The model under review builds one solid part; all positions refer to its coordinate system, in mm. A direction names the side the tool comes from. Give positions to 0.01 mm unless a question says otherwise; leave off trailing zeros. Loops run counter-clockwise (first coordinate to the right, second up) from the corner with the lowest first, then second, coordinate; pieces in that order, holes last. Notation, with made-up numbers: M -15.5,-24 L 13.5,-24 A18 cw 13.5,-17 Z; hole C -24,32.25 d7. An arc over 180 degrees is marked long. Return JSON: item names as keys, results as strings.
```python
from build123d import *

# Parameters (mm, degrees)
SKETCH1_W           = 320
SKETCH1_H           = 82.5
BOSS_EXTRUDE1_DEPTH = 43.48
SKETCH3_W           = 20
SKETCH3_H           = 20
CUT_EXTRUDE1_DEPTH  = 15
SKETCH5_W           = 320
SKETCH5_H           = 82.5
BOSS_EXTRUDE3_DEPTH = 5


with BuildPart() as part:
    # Sketch1 → Boss-Extrude1 (new body)
    with BuildSketch(Plane(origin=(0, 0, 0), x_dir=(1, 0, 0), z_dir=(0, 1, 0))):
        Rectangle(SKETCH1_W, SKETCH1_H)
        Polygon((-135, 30), (-115, 30), (-115, 7.5), (-10, 7.5), (-10, 30), (10, 30), (10, 7.5), (115, 7.5), (115, 30), (135, 30), (135, -30), (115, -30), (115, -7.5), (10, -7.5), (10, -30), (-10, -30), (-10, -7.5), (-115, -7.5), (-115, -30), (-135, -30), align=None, mode=Mode.SUBTRACT)
    extrude(amount=-BOSS_EXTRUDE1_DEPTH)

    # Sketch3 → Cut-Extrude1 (cut)
    with BuildSketch(Plane.XY.offset(41.25)):
        with Locations((0, -33.48)):
            Rectangle(SKETCH3_W, SKETCH3_H)
        with Locations((125, -33.48)):
            Rectangle(SKETCH3_W, SKETCH3_H)
        with Locations((-125, -33.48)):
            Rectangle(SKETCH3_W, SKETCH3_H)
    extrude(amount=-CUT_EXTRUDE1_DEPTH, mode=Mode.SUBTRACT)

    # Sketch5 → Boss-Extrude3 (add)
    with BuildSketch(Plane.XZ.offset(43.48)):
        Rectangle(SKETCH5_W, SKETCH5_H)
    extrude(amount=BOSS_EXTRUDE3_DEPTH)


solid = part.part
```
1) Consider section A-A on y = -38.5. Write out the cut boundary in (x, z).
From the geometry:
{"outline": "M -160,-41.25 L 160,-41.25 L 160,41.25 L 135,41.25 L 135,-30 L 115,-30 L 115,-7.5 L 10,-7.5 L 10,-30 L -10,-30 L -10,-7.5 L -115,-7.5 L -115,-30 L -135,-30 L -135,41.25 L -160,41.25 Z; M -115,7.5 L -10,7.5 L -10,41.25 L -115,41.25 Z; M 10,7.5 L 115,7.5 L 115,41.25 L 10,41.25 Z"}
2) Consider section C-C on x = 4.5. Write out the cut boundary in (y, z), then the cut area to 3 significant figures.
From the geometry:
{"outline": "M -48.48,-41.25 L 0,-41.25 L 0,-30 L -43.48,-30 L -43.48,41.25 L -48.48,41.25 Z; M -23.48,30 L 0,30 L 0,41.25 L -23.48,41.25 Z", "area": "1,170 mm²"}
3) Insertion check: pin 1 (6 mm diameter, centred on x = -5, y = -25.5, fed in from +Z). The pin has a flat end and moves straight along its axis. Give the tip position at first contact, or say it passes through.
From the geometry:
{"pin 1": "z = 41.25"}
4) Wall thickness on L1, parallel to X at y = -34, z = 9; L2, parallel to Z at x = -78, y = -21.5; L3, parallel to X at y = -32, z = -1: over which ranges is each line inside the solid? List them lowest first. Write a range as from..to.
From the geometry:
{"L1": "-160..-135, -115..-10, 10..115, 135..160", "L2": "-41.25..-7.5, 7.5..41.25", "L3": "-160..-135, 135..160"}
5) Consider section B-B on x = 41. Write out the cut boundary in (y, z), then the cut area to 3 significant figures.
From the geometry:
{"outline": "M -48.48,-41.25 L 0,-41.25 L 0,-7.5 L -43.48,-7.5 L -43.48,7.5 L 0,7.5 L 0,41.25 L -48.48,41.25 Z", "area": "3,350 mm²"}
6) The part is to be moulded in two halves that separate along Y. For faces 1 (the face through (-2, 0, -37)), 2 (the face through (125, -12, 30)), 3 (the face through (115, -22, 21)), say which applies: released by +Y, released by -Y, zero draft, split by the parting line, or undercut.
From the geometry:
{"face 1": "released by +Y", "face 2": "zero draft", "face 3": "undercut"}
7) Tool access review of faces 4 (the face through (125, -23.48, 36)), 5 (the face through (-10, -22, 21)), 6 (the face through (-125, -12, 30)), 7 (the face through (-2, -48.48, 1)): name each direction out of +Z, -Z, +X, -X, +Y, -Y from which nothing blocks a thin tool from reaching the whole face with its end or side.
From the geometry:
{"face 4": "+Z", "face 5": "none", "face 6": "+Y", "face 7": "+Z, -Z, +X, -X, -Y"}
8) Consider section D-D on z = -0.5. Write out the cut boundary in (x, y), then the cut area to 3 significant figures.
From the geometry:
{"outline": "M -160,-48.48 L 160,-48.48 L 160,0 L 135,0 L 135,-43.48 L -135,-43.48 L -135,0 L -160,0 Z", "area": "3,770 mm²"}
